```python
from build123d import *

# Parameters (mm, degrees)
F0_W     = 4
F0_H     = 3
F1_DEPTH = 0.15
F2_DEPTH = 1.9
F3_W     = 0.15
F3_H     = 7
F4_DEPTH = 8
F6_DEPTH = 25
F7_R     = 0.5


with BuildPart() as f1:
    # F0 (on Top) → F1 (new body)
    with BuildSketch(Plane.XY):
        with BuildLine():
            Line((96.425, -0.5), (96.425, -3.5))
            Line((96.425, -3.5), (100.425, -3.5))
            Line((100.425, -3.5), (110.2, -3.5))
            Line((110.2, -3.5), (123.975, -3.5))
            Line((123.975, -3.5), (123.975, -0.5))
            Line((123.975, -0.5), (119.375, -0.5))
            ThreePointArc((119.375, -0.5), (119.0921572875, -0.3828427125), (118.975, -0.1))
            Line((118.975, -0.1), (118.975, 0.1))
            ThreePointArc((118.975, 0.1), (119.0921572875, 0.3828427125), (119.375, 0.5))
            Line((119.375, 0.5), (123.975, 0.5))
            Line((123.975, 0.5), (123.975, 3.5))
            Line((123.975, 3.5), (110.2, 3.5))
            Line((110.2, 3.5), (100.425, 3.5))
            Line((100.425, 3.5), (96.425, 3.5))
            Line((96.425, 3.5), (96.425, 0.5))
            Line((96.425, 0.5), (101.025, 0.5))
            ThreePointArc((101.025, 0.5), (101.3078427125, 0.3828427125), (101.425, 0.1))
            Line((101.425, 0.1), (101.425, -0.1))
            ThreePointArc((101.425, -0.1), (101.3078427125, -0.3828427125), (101.025, -0.5))
            Line((101.025, -0.5), (96.425, -0.5))
        make_face()
        with BuildLine():
            Line((13.775, -0.5), (13.775, -3.5))
            Line((13.775, -3.5), (27.55, -3.5))
            Line((27.55, -3.5), (41.325, -3.5))
            Line((41.325, -3.5), (41.325, -0.5))
            Line((41.325, -0.5), (36.725, -0.5))
            ThreePointArc((36.725, -0.5), (36.4421572875, -0.3828427125), (36.325, -0.1))
            Line((36.325, -0.1), (36.325, 0.1))
            ThreePointArc((36.325, 0.1), (36.4421572875, 0.3828427125), (36.725, 0.5))
            Line((36.725, 0.5), (41.325, 0.5))
            Line((41.325, 0.5), (41.325, 3.5))
            Line((41.325, 3.5), (27.55, 3.5))
            Line((27.55, 3.5), (13.775, 3.5))
            Line((13.775, 3.5), (13.775, 0.5))
            Line((13.775, 0.5), (18.375, 0.5))
            ThreePointArc((18.375, 0.5), (18.6578427125, 0.3828427125), (18.775, 0.1))
            Line((18.775, 0.1), (18.775, -0.1))
            ThreePointArc((18.775, -0.1), (18.6578427125, -0.3828427125), (18.375, -0.5))
            Line((18.375, -0.5), (13.775, -0.5))
        make_face()
        with BuildLine():
            Line((41.325, -0.5), (41.325, -3.5))
            Line((41.325, -3.5), (55.1, -3.5))
            Line((55.1, -3.5), (68.875, -3.5))
            Line((68.875, -3.5), (68.875, -0.5))
            Line((68.875, -0.5), (64.275, -0.5))
            ThreePointArc((64.275, -0.5), (63.9921572875, -0.3828427125), (63.875, -0.1))
            Line((63.875, -0.1), (63.875, 0.1))
            ThreePointArc((63.875, 0.1), (63.9921572875, 0.3828427125), (64.275, 0.5))
            Line((64.275, 0.5), (68.875, 0.5))
            Line((68.875, 0.5), (68.875, 3.5))
            Line((68.875, 3.5), (55.1, 3.5))
            Line((55.1, 3.5), (41.325, 3.5))
            Line((41.325, 3.5), (41.325, 0.5))
            Line((41.325, 0.5), (45.925, 0.5))
            ThreePointArc((45.925, 0.5), (46.2078427125, 0.3828427125), (46.325, 0.1))
            Line((46.325, 0.1), (46.325, -0.1))
            ThreePointArc((46.325, -0.1), (46.2078427125, -0.3828427125), (45.925, -0.5))
            Line((45.925, -0.5), (41.325, -0.5))
        make_face()
        with BuildLine():
            Line((68.875, -0.5), (68.875, -3.5))
            Line((68.875, -3.5), (82.65, -3.5))
            Line((82.65, -3.5), (96.425, -3.5))
            Line((96.425, -3.5), (96.425, -0.5))
            Line((96.425, -0.5), (91.825, -0.5))
            ThreePointArc((91.825, -0.5), (91.5421572875, -0.3828427125), (91.425, -0.1))
            Line((91.425, -0.1), (91.425, 0.1))
            ThreePointArc((91.425, 0.1), (91.5421572875, 0.3828427125), (91.825, 0.5))
            Line((91.825, 0.5), (96.425, 0.5))
            Line((96.425, 0.5), (96.425, 3.5))
            Line((96.425, 3.5), (82.65, 3.5))
            Line((82.65, 3.5), (68.875, 3.5))
            Line((68.875, 3.5), (68.875, 0.5))
            Line((68.875, 0.5), (73.475, 0.5))
            ThreePointArc((73.475, 0.5), (73.7578427125, 0.3828427125), (73.875, 0.1))
            Line((73.875, 0.1), (73.875, -0.1))
            ThreePointArc((73.875, -0.1), (73.7578427125, -0.3828427125), (73.475, -0.5))
            Line((73.475, -0.5), (68.875, -0.5))
        make_face()
        with BuildLine():
            Line((0, 3.5), (0, -3.5))
            Line((0, -3.5), (13.775, -3.5))
            Line((13.775, -3.5), (13.775, -0.5))
            Line((13.775, -0.5), (9.175, -0.5))
            ThreePointArc((9.175, -0.5), (8.8921572875, -0.3828427125), (8.775, -0.1))
            Line((8.775, -0.1), (8.775, 0.1))
            ThreePointArc((8.775, 0.1), (8.8921572875, 0.3828427125), (9.175, 0.5))
            Line((9.175, 0.5), (13.775, 0.5))
            Line((13.775, 0.5), (13.775, 3.5))
            Line((13.775, 3.5), (0, 3.5))
        make_face()
        with Locations((125.975, -2)):
            Rectangle(F0_W, F0_H)
        with Locations((125.975, 2)):
            Rectangle(F0_W, F0_H)
    extrude(amount=F1_DEPTH)

    # F2 (add): a face of the model
    f2_faces = [f1.faces().sort_by_distance(p)[0] for p in [
        (0, 0, 0.075),
    ]]
    extrude(f2_faces, amount=F2_DEPTH)

    # F3 (on face) → F4 (join)
    with BuildSketch(Plane(origin=(0, 0, 0), x_dir=(1, 0, 0), z_dir=(0, 0, -1))):
        with Locations((-1.825, 0)):
            Rectangle(F3_W, F3_H)
    extrude(amount=F4_DEPTH)

    # F5 (on face) → F6 (cut)
    with BuildSketch(Plane(origin=(-1.9, 0, 0), x_dir=(0, -1, 0), z_dir=(-1, 0, 0))):
        with BuildLine():
            ThreePointArc((1.4, -7.1), (1.1363961031, -7.7363961031), (0.5, -8))
            Line((0.5, -8), (3.5, -8))
            Line((3.5, -8), (3.5, -0.8))
            ThreePointArc((3.5, -0.8), (3.4707106781, -0.8707106781), (3.4, -0.9))
            Line((3.4, -0.9), (2.3, -0.9))
            ThreePointArc((2.3, -0.9), (1.6636038969, -1.1636038969), (1.4, -1.8))
            Line((1.4, -1.8), (1.4, -7.1))
        make_face()
        with BuildLine():
            Line((-3.5, -8), (-0.5, -8))
            ThreePointArc((-0.5, -8), (-1.1363961031, -7.7363961031), (-1.4, -7.1))
            Line((-1.4, -7.1), (-1.4, -1.8))
            ThreePointArc((-1.4, -1.8), (-1.6636038969, -1.1636038969), (-2.3, -0.9))
            Line((-2.3, -0.9), (-3.4, -0.9))
            ThreePointArc((-3.4, -0.9), (-3.4707106781, -0.8707106781), (-3.5, -0.8))
            Line((-3.5, -0.8), (-3.5, -8))
        make_face()
        with BuildLine():
            ThreePointArc((-0.45, -4.7), (0, -5.15), (0.45, -4.7))
            ThreePointArc((0.45, -4.7), (0, -4.25), (-0.45, -4.7))
        make_face()
        with BuildLine():
            ThreePointArc((-0.45, -6.6), (0, -6.15), (0.45, -6.6))
            Line((0.45, -6.6), (0.45, -4.7))
            ThreePointArc((0.45, -4.7), (0, -5.15), (-0.45, -4.7))
            Line((-0.45, -4.7), (-0.45, -6.6))
        make_face()
        with BuildLine():
            ThreePointArc((-0.45, -6.6), (0, -7.05), (0.45, -6.6))
            ThreePointArc((0.45, -6.6), (0, -6.15), (-0.45, -6.6))
        make_face()
    extrude(amount=-F6_DEPTH, mode=Mode.SUBTRACT)

    # F7
    f7_edges = [f1.edges().sort_by_distance(p)[0] for p in [
        (-1.9, 0, 0.15),
        (-1.75, 0, 0),
    ]]
    fillet(f7_edges, radius=F7_R)


solid = f1.part
```
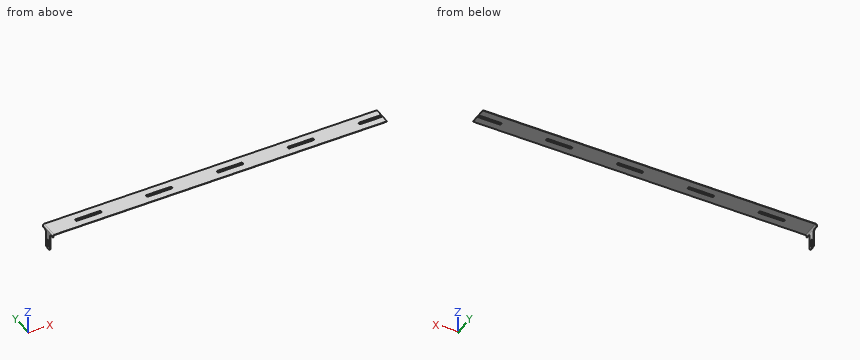
Check sheet for the modelled part. Datum: model origin and axes. Units: mm. Round coordinates to 2 decimals unless told otherwise and drop trailing zeros. Loops run counter-clockwise (first coordinate to the right, second up) from the corner with the lowest first, then second, coordinate; pieces in that order, holes last. Notation, with made-up numbers: (10, 28) -> (31, 28) arc R22 cw to (31, 56) -> close; hole circle Ø7 at (80, 9). An arc over 180 degrees is marked (long way). Write item = value, one per line. Start each with the question number.
1) Gauge pin test, flat ends, axial feed: pin 1 Ø2 at (x, y) = (31, -0.5) entering from -Z; pin 2 Ø3 at (x, z) = (47, -1) entering from +Y. Record the tip position at first contact, or that the pin passes through.
2) Sectioned sample at A-A, the plane x = 43.5. Record the cut outline in (y, z), plus the area to 3 significant figures.
3) Sectioned sample at B-B, the plane x = 87. Record the cut outline in (y, z).
4) Thickness scan on probe 1 along Z at (x, y) = (91, -0.5). Record the ranges inside material, lowest first.
Results are:
q1.pin_1 = 0
q1.pin_2 = 3.5
q2.outline = (-3.5, 0) -> (-0.5, 0) -> (-0.5, 0.15) -> (-3.5, 0.15) -> close; (0.5, 0) -> (3.5, 0) -> (3.5, 0.15) -> (0.5, 0.15) -> close
q2.area = 0.900 mm^2
q3.outline = (-3.5, 0) -> (3.5, 0) -> (3.5, 0.15) -> (-3.5, 0.15) -> close
q4.probe_1 = 0 to 0.15
